Geometry check sheet. Reference: drawing and pictorial views, mm from the part's lowest x, y, z. Give positions to 0.01 mm unless a question says otherwise; leave off trailing zeros. Order: outer loops, then holes, each group sorted by start corner. A loop starts at its lowest first (then second) coordinate and runs counter-clockwise, first axis right, second up. Notation, with made-up numbers: (36, 82.25) - (80, 82.25) arc R28 ccw to (80, 119.25) - close; hole circle Ø2 at (88.25, 63). An arc over 180 degrees is marked (long way). Answer as a JSON object with one key per item and string values.
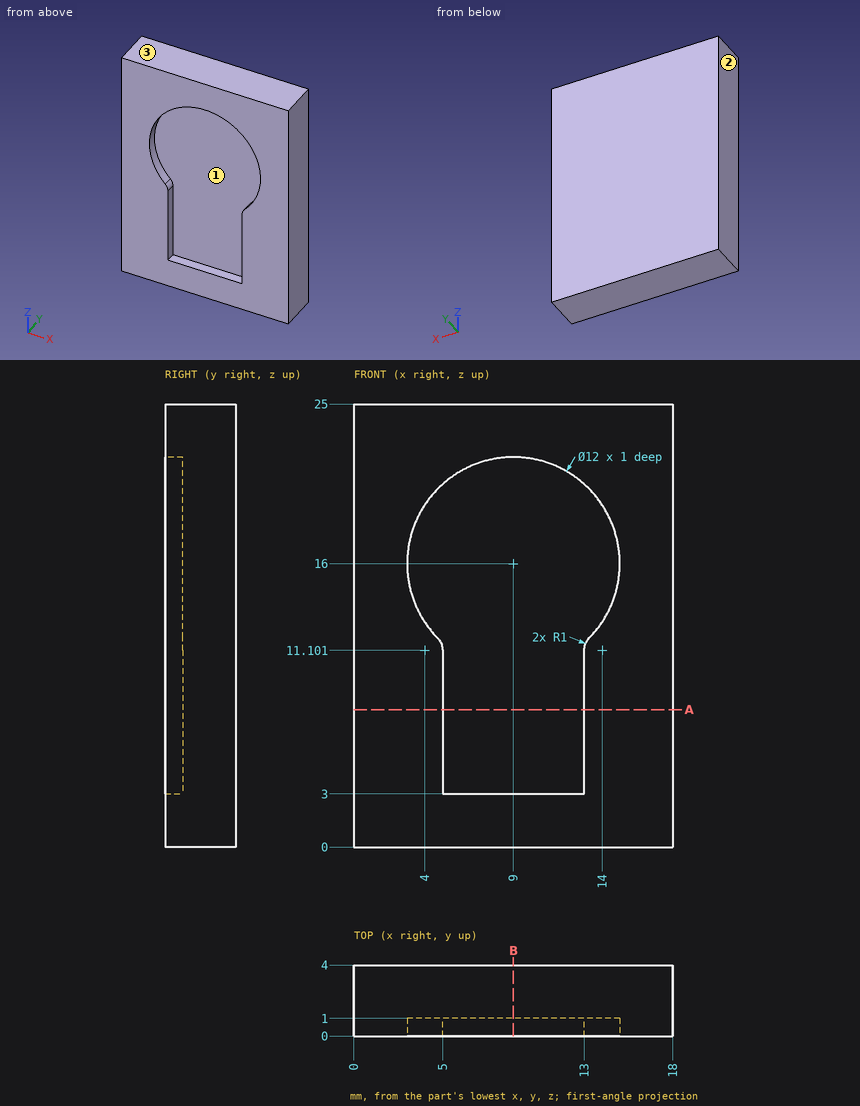
(1) Section check A-A (z = 7.75). Record the cut outline in (x, y), then the cut area to 3 significant figures.
Computed values:
{"outline": "(0, 0) - (5, 0) - (5, 1) - (13, 1) - (13, 0) - (18, 0) - (18, 4) - (0, 4) - close", "area": "64.0 mm²"}
(2) Gauge pin test, flat end, axial feed: pin 1 Ø1.5 at (y, z) = (0.5, 12) entering from -X. Record the tip position at first contact, or that the pin passes through.
Computed values:
{"pin 1": "stops at x = 0"}
(3) Material ranges on line 1 along Z through (x, y) = (9, 0.4); line 2 along X through (y, z) = (0.55, 16.25); line 3 along Y through (x, z) = (11, 13), recorded low to high. Write a range as [from, to].
Computed values:
{"line 1": "z = [0, 3], [22, 25]", "line 2": "x = [0, 3.01], [14.99, 18]", "line 3": "y = [1, 4]"}
(4) Release check for a two-part mould opening along X. For the marked faces 1, 2 and 3 record: pulls with the +X half, pulls with the -X half, needs draft (parallel to the pull), parting line crosses it, or undercut.
Computed values:
{"face 1": "undercut", "face 2": "pulls with the -X half", "face 3": "needs draft"}
(5) Section check B-B (x = 9). Record the cut outline in (y, z).
Computed values:
{"outline": "(0, 0) - (4, 0) - (4, 25) - (0, 25) - (0, 22) - (1, 22) - (1, 3) - (0, 3) - close"}
